The model under review builds one solid part; all positions refer to its coordinate system, in mm. A direction names the side the tool comes from. Coordinates: 2 decimals unless noted, no trailing zeros. Order: outer loops, then holes, each group sorted by start corner. A loop starts at its lowest first (then second) coordinate and runs counter-clockwise, first axis right, second up. Notation, with made-up numbers: (32.5, 36) - (90.5, 36) arc R17 cw to (90.5, 58) - close; hole circle Ø11 at (45, 63.5). An arc over 180 degrees is marked (long way). Answer in a Markdown table with one row per item.
```python
from build123d import *

# Parameters (mm, degrees)
SKETCH_R     = 1.3
SKETCH_W     = 14
SKETCH_H     = 12
PAD_DEPTH    = 3
FILLET_R     = 0.75
POCKET_DEPTH = 5
FILLET001_R  = 0.5
CHAMFER_SIZE = 1
PAD001_DEPTH = 3
FILLET002_R  = 2
SKETCH004_W  = 0.400118
SKETCH004_H  = 2.725121
PAD002_DEPTH = 0.2


with BuildPart() as part:
    # Sketch (on XY_Plane of Origin) → Pad (new body)
    with BuildSketch(Plane.XY):
        Polygon((-9.75, -9.75), (9.75, -9.75), (9.75, 9.75), (-9.75, 9.75), (-21, 9.75), (-21, -0.75), (-21.75, -0.75), (-29.75, -2.75), (-29.75, -3.75), (-3, -3.75), (-3, -5.75), (-29.75, -5.75), (-29.75, -6.75), (-21.75, -9.75), align=None)
        with Locations((0, 6)):
            Circle(SKETCH_R, mode=Mode.SUBTRACT)
        with Locations((0, -6)):
            Circle(SKETCH_R, mode=Mode.SUBTRACT)
        with Locations((-10, 3)):
            Rectangle(SKETCH_W, SKETCH_H, mode=Mode.SUBTRACT)
    extrude(amount=PAD_DEPTH)

    # Fillet
    fillet_edges = [part.edges().sort_by_distance(p)[0] for p in [
        (-3, -3, 1.5),
        (-3, 9, 1.5),
        (-17, 9, 1.5),
        (-17, -3, 1.5),
        (-3, -3.75, 1.5),
        (-3, -5.75, 1.5),
    ]]
    fillet(fillet_edges, radius=FILLET_R)

    # Sketch002 (on Face26 of Fillet) → Pocket (cut)
    with BuildSketch(Plane.XY.offset(3)):
        with BuildLine():
            ThreePointArc((-18.4, -9.353833), (-19, -8.753833), (-19.6, -9.353833))
            Line((-19.6, -9.353833), (-19.6, -11.103725))
            ThreePointArc((-19.6, -11.103725), (-19, -11.703725), (-18.4, -11.103725))
            Line((-18.4, -9.353833), (-18.4, -11.103725))
        make_face()
        with BuildLine():
            ThreePointArc((-18.4, 12.382466), (-19, 12.982466), (-19.6, 12.382466))
            Line((-19.6, 12.382466), (-19.6, 9.326973))
            ThreePointArc((-19.6, 9.326973), (-19, 8.726973), (-18.4, 9.326973))
            Line((-18.4, 12.382466), (-18.4, 9.326973))
        make_face()
    extrude(amount=-POCKET_DEPTH, mode=Mode.SUBTRACT)

    # Fillet001
    fillet001_edges = [part.edges().sort_by_distance(p)[0] for p in [
        (-21, 9.75, 1.5),
        (-21, -0.75, 1.5),
        (9.75, -9.75, 1.5),
        (9.75, 9.75, 1.5),
        (-19.6, 9.75, 1.5),
        (-18.4, 9.75, 1.5),
        (-19.6, -9.75, 1.5),
        (-18.4, -9.75, 1.5),
        (-29.75, -6.75, 1.5),
        (-29.75, -2.75, 1.5),
    ]]
    fillet(fillet001_edges, radius=FILLET001_R)

    # Chamfer
    chamfer_edges = [part.edges().sort_by_distance(p)[0] for p in [
        (-1.3, 6, 3),
        (-1.3, -6, 3),
    ]]
    chamfer(chamfer_edges, length=CHAMFER_SIZE)

    # Sketch003 (on Face4 of Chamfer) → Pad001 (join)
    with BuildSketch(Plane.XY.offset(3)):
        Polygon((-14.75, 9), (-13.017949, 8), (-6.982051, 8), (-5.25, 9), align=None)
        Polygon((-14.75, -3), (-13.017949, -2), (-6.982051, -2), (-5.25, -3), align=None)
    extrude(amount=-PAD001_DEPTH)

    # Fillet002
    fillet002_edges = [part.edges().sort_by_distance(p)[0] for p in [
        (-5.25, -3, 1.5),
        (-14.75, -3, 1.5),
        (-13.017949, -2, 1.5),
        (-6.982051, -2, 1.5),
        (-5.25, 9, 1.5),
        (-6.982051, 8, 1.5),
        (-13.017949, 8, 1.5),
        (-14.75, 9, 1.5),
    ]]
    fillet(fillet002_edges, radius=FILLET002_R)

    # Sketch004 (on Face1 of Fillet002) → Pad002 (join)
    with BuildSketch(Plane(origin=(0, 0, 0), x_dir=(1, 0, 0), z_dir=(0, 0, -1))):
        with Locations((-25.583762, 4.610938)):
            Rectangle(SKETCH004_W, SKETCH004_H)
    extrude(amount=-PAD002_DEPTH)


solid = part.part
```
Item 1: We need section D-D, the plane x = -19. Write out the cut boundary in (y, z), then the cut area to 3 significant figures.
Check values:
| item | result |
|---|---|
| outline | (-8.75, 0) - (-5.75, 0) - (-5.75, 3) - (-8.75, 3) - close; (-3.75, 0) - (8.73, 0) - (8.73, 3) - (-3.75, 3) - close |
| area | 46.4 mm^2 |
Item 2: Clearance check with flat-ended pins moving along their axes: pin 1 Ø1.5 at (y, z) = (3, 1.5) entering from -X; pin 2 Ø1.6 at (x, y) = (0, -6) entering from -Z; pin 3 Ø5 at (x, y) = (-16, -1.5) entering from +Z. State where each tip first meets the part, or that it passes through.
Check values:
| item | result |
|---|---|
| pin 1 | x = -21 |
| pin 2 | through |
| pin 3 | z = 3 |
Item 3: Tool access review of faces 4 (the face through (-25.64, -8.29, 1.48)), 5 (the face through (-3, 3, 1)): name each direction out of +Z, -Z, +X, -X, +Y, -Y from which nothing blocks a thin tool from reaching the whole face with its end or side.
Check values:
| item | result |
|---|---|
| face 4 | +Z, -Z, -X, -Y |
| face 5 | +Z, -Z |
Item 4: We need section A-A, the plane x = 0. Write out the cut boundary in (y, z).
Check values:
| item | result |
|---|---|
| outline | (-9.75, 0) - (-7.3, 0) - (-7.3, 2) - (-8.3, 3) - (-9.75, 3) - close; (-4.7, 0) - (4.7, 0) - (4.7, 2) - (3.7, 3) - (-3.7, 3) - (-4.7, 2) - close; (7.3, 0) - (9.75, 0) - (9.75, 3) - (8.3, 3) - (7.3, 2) - close |
Item 5: To check wall thickness, follow line 1 (Y direction, x = 0, z = 1.45); line 2 (Y direction, x = -10.5, z = 2.05); line 3 (X direction, y = 7.75, z = 1.1). State the ranges of each line that lie inside material, in increasing order. Write a range as from..to.
Check values:
| item | result |
|---|---|
| line 1 | -9.75..-7.3, -4.7..4.7, 7.3..9.75 |
| line 2 | -9.75..-5.75, -3.75..-2, 8..9.75 |
| line 3 | -21..-17, -3..9.75 |
Item 6: We need section B-B, the plane y = 0.75. Write out the cut boundary in (x, z).
Check values:
| item | result |
|---|---|
| outline | (-21, 0) - (-17, 0) - (-17, 3) - (-21, 3) - close; (-3, 0) - (9.75, 0) - (9.75, 3) - (-3, 3) - close |
Item 7: Mouldability with a two-part tool opening along Y and no side actions: class faces 1 (the face through (-21, 5, 1)), 2 (the face through (-17, -5.75, 1)), 3 (the face through (-25.51, -1.69, 1.48)) as +Y half, -Y half, draft (parallel to the pull), parting line (faces both ways), or undercut.
Check values:
| item | result |
|---|---|
| face 1 | draft |
| face 2 | undercut |
| face 3 | +Y half |
Item 8: We need section C-C, the plane y = 6. Write out the cut boundary in (x, z), then the cut area to 4 significant figures.
Check values:
| item | result |
|---|---|
| outline | (-21, 0) - (-17, 0) - (-17, 3) - (-21, 3) - close; (-3, 0) - (-1.3, 0) - (-1.3, 2) - (-2.3, 3) - (-3, 3) - close; (1.3, 0) - (9.75, 0) - (9.75, 3) - (2.3, 3) - (1.3, 2) - close |
| area | 41.45 mm^2 |
